```python
from build123d import *

# Parameters (mm, degrees)
F1_DEPTH      = 63.5
F1_DEPTH_BACK = 63.5
F2_DEPTH      = 12.7
F2_DEPTH_BACK = 12.7


with BuildPart() as f1:
    # F0 (on Front) → F1 (new body, two sides)
    with BuildSketch(Plane.XZ) as f1_sk:
        Polygon((5.371508698, -65.522043058), (5.371508698, 97.9658832341), (-6.8627363071, 97.9658832341), (-6.8627363071, 48.6798776739), (-6.8627363071, 40.9828163683), (-6.8627363071, 9.4113918418), (-6.8627363071, 0), (-6.8627363071, -12.8354746848), (-6.8627363071, -27.4818117807), (-6.8627363071, -65.522043058), (-58.128491302, -65.522043058), (-58.128491302, -79.8341167659), (-6.8627363071, -79.8341167659), (5.371508698, -79.8341167659), align=None)
    extrude(amount=F1_DEPTH)
    extrude(f1_sk.sketch, amount=-F1_DEPTH_BACK)

    # F0 (on Front) → F2 (join, two sides)
    with BuildSketch(Plane.XZ) as f2_sk:
        with BuildLine():
            Line((-6.8627363071, 40.9828163683), (-6.8627363071, 48.6798776739))
            Line((-6.8627363071, 48.6798776739), (-33.0135776846, 48.6798776739))
            ThreePointArc((-33.0135776846, 48.6798776739), (-41.8657904366, 74.1654240795), (-44.0332744745, 47.2734780892))
            Line((-44.0332744745, 47.2734780892), (-50.8055312902, 10.6125895488))
            ThreePointArc((-50.8055312902, 10.6125895488), (-47.911326645, 4.8382984922), (-43.1451888861, 9.1975172982))
            Line((-43.1451888861, 9.1975172982), (-38.6480391026, 33.7588861585))
            Line((-38.6480391026, 33.7588861585), (-30.8785432337, 9.1975172982))
            Line((-30.8785432337, 9.1975172982), (-6.8627363071, -27.4818117807))
            Line((-6.8627363071, -27.4818117807), (-6.8627363071, -12.8354746848))
            Line((-6.8627363071, -12.8354746848), (-21.3106013834, 9.1975172982))
            Line((-21.3106013834, 9.1975172982), (-15.6995095313, 9.2722494155))
            Line((-15.6995095313, 9.2722494155), (-6.8627363071, 0))
            Line((-6.8627363071, 0), (-6.8627363071, 9.4113918418))
            Line((-6.8627363071, 9.4113918418), (-13.6101442425, 17.1438418329))
            Line((-13.6101442425, 17.1438418329), (-21.6717980802, 17.1438418329))
            Line((-21.6717980802, 17.1438418329), (-29.3174761241, 40.9828163683))
            Line((-29.3174761241, 40.9828163683), (-6.8627363071, 40.9828163683))
        make_face()
        with BuildLine():
            ThreePointArc((-48.0739454946, 58.0599678974), (-50.4266953443, 59.1407090556), (-52.635530327, 60.4914426804))
            ThreePointArc((-52.635530327, 60.4914426804), (-50.3327931811, 62.4139887897), (-47.7398221818, 63.9223930132))
            add(Edge.make_bspline(
                [(-47.7398221818, 63.9223930132), (-48.8867841974, 61.1721295429), (-48.0739454946, 58.0599678975)],
                knots=[4.0684612213, 4.0684612213, 4.0684612213, 5.1518534756, 5.1518534756, 5.1518534756], degree=2, weights=[1, 0.856835408, 1]))
        make_face(mode=Mode.SUBTRACT)
        with BuildLine():
            ThreePointArc((-37.4315397632, 56.7311223598), (-40.1206351817, 56.5654747777), (-42.8097306001, 56.7311223598))
            add(Edge.make_bspline(
                [(-42.8097306001, 56.7311223598), (-40.3777204819, 61.7412384639), (-43.4961171085, 65.3130386577)],
                knots=[0.8526714179, 0.8526714179, 0.8526714179, 2.5748864382, 2.5748864382, 2.5748864382], degree=2, weights=[1, 0.6515977499, 1]))
            ThreePointArc((-43.4961171085, 65.3130386577), (-40.1206351817, 65.6361303431), (-36.7451532548, 65.3130386577))
            add(Edge.make_bspline(
                [(-36.7451532548, 65.3130386577), (-39.8635498815, 61.7412384639), (-37.4315397632, 56.7311223598)],
                knots=[0.5667062154, 0.5667062154, 0.5667062154, 2.2889212357, 2.2889212357, 2.2889212357], degree=2, weights=[1, 0.6515977499, 1]))
        make_face(mode=Mode.SUBTRACT)
        with BuildLine():
            ThreePointArc((-32.5014481816, 63.9223930132), (-29.9084771822, 62.4139887897), (-27.6057400363, 60.4914426804))
            ThreePointArc((-27.6057400363, 60.4914426804), (-29.8145750191, 59.1407090556), (-32.1673248687, 58.0599678974))
            add(Edge.make_bspline(
                [(-32.1673248687, 58.0599678975), (-31.3544861659, 61.1721295429), (-32.5014481816, 63.9223930132)],
                knots=[4.2729244852, 4.2729244852, 4.2729244852, 5.3563167394, 5.3563167394, 5.3563167394], degree=2, weights=[1, 0.856835408, 1]))
        make_face(mode=Mode.SUBTRACT)
    extrude(amount=F2_DEPTH)
    extrude(f2_sk.sketch, amount=-F2_DEPTH_BACK)


solid = f1.part
```
Part model, mm, in its own coordinate system. A direction names the side the tool comes from. Round coordinates to 2 decimals unless told otherwise and drop trailing zeros. Write each loop counter-clockwise with the first axis right and the second up, starting at its lowest first coordinate (ties: lowest second). Pieces come first, ordered by that corner, then holes.
Item 1: Cut at B-B, the plane y = 55.5. Give the cut face in (x, z), plus the area to 3 significant figures.
Results:
outline: (-58.13, -79.83) - (5.37, -79.83) - (5.37, 97.97) - (-6.86, 97.97) - (-6.86, -65.52) - (-58.13, -65.52) - close
area: 2,910 mm2
Item 2: Which spindle directions (+Z, -Z, +X, -X, +Y, -Y) get a long thin tool onto all of the face, cutting with end or side? Do faces 5 (the flat face through (-58.128, -1, -73)), 6 (the flat face through (-20, 0, 48.68)). Say none if no direction does.
Results:
face 5: +Z, -Z, -X, +Y, -Y
face 6: +Y, -Y
Item 3: Cut at A-A, the plane z = 28.5. Give the cut face in (x, y), plus the area to 3 significant figures.
Results:
outline: (-47.5, -12.7) - (-39.61, -12.7) - (-39.61, 12.7) - (-47.5, 12.7) - close; (-36.98, -12.7) - (-25.31, -12.7) - (-25.31, 12.7) - (-36.98, 12.7) - close; (-6.86, -63.5) - (5.37, -63.5) - (5.37, 63.5) - (-6.86, 63.5) - close
area: 2,050 mm2
Item 4: Probe L1, parallel to X at y = -17.5, z = -20; L2, parallel to Z at x = -19, y = 6; L3, parallel to Y at x = -36, z = 29.5. List the from-to ranges inside material, lowest first.
Results:
L1: x = -6.86 to 5.37
L2: z = -79.83 to -65.52, -8.94 to 5.67, 9.23 to 17.14, 40.98 to 48.68
L3: y = -12.7 to 12.7
Item 5: Cut at D-D, the plane y = -5. Count the separate pieces of the cut face and the enclosed holes in it, plus the area to 3 significant figures.
Results:
separate pieces: 1
enclosed holes: 5
area: 4,750 mm2
Item 6: Cut at C-C, the plane z = 2. Give the cut face in (x, y), plus the area to 3 significant figures.
Results:
outline: (-26.17, -12.7) - (-16.59, -12.7) - (-16.59, 12.7) - (-26.17, 12.7) - close; (-8.77, -12.7) - (-6.86, -12.7) - (-6.86, -63.5) - (5.37, -63.5) - (5.37, 63.5) - (-6.86, 63.5) - (-6.86, 12.7) - (-8.77, 12.7) - close
area: 1,850 mm2
Item 7: Drop flat-ended pins along their axis: pin 1 Ø15.5 at (x, y) = (-25.5, -7) entering from +Z; pin 2 Ø1.5 at (y, z) = (27, 11.5) entering from -X; pin 3 Ø5 at (x, y) = (-14.5, -5) entering from +Z. Give the stop position or say it passes through.
Results:
pin 1: stops at z = 72.44
pin 2: stops at x = -6.86
pin 3: stops at z = 48.68
Item 8: Two-plate mould, pull along X, no slides. Class faces 1 (the cylindrical face through (-48.014, -0.178, 4.859)), 2 (the cylindrical face through (-41.343, -0.178, 74.222)), 3 (the flat face through (-47.37, -0.18, 29.2)), 4 (the flat face through (-31, 12.7, 35)): +X half, -X half, draft (parallel to the pull), parting line (faces both ways), or undercut.
Results:
face 1: undercut
face 2: undercut
face 3: -X half
face 4: draft
